```python
from build123d import *

# Parameters (mm, degrees)
F0_W     = 127
F0_H     = 76.2
F1_DEPTH = 50.8
F2_R     = 7.62
F3_W     = 7
F3_H     = 15.2537040412
F4_DEPTH = 16.4084
F4_TAPER = -3
F5_W     = 5
F5_H     = 4.0000001475
F6_DEPTH = 11.938
F6_TAPER = -3


with BuildPart() as f1:
    # F0 (on Front) → F1 (new body)
    with BuildSketch(Plane.XZ):
        Rectangle(F0_W, F0_H)
    extrude(amount=F1_DEPTH)

    # F2
    f2_edges = [f1.edges().sort_by_distance(p)[0] for p in [
        (0, -50.8, 38.1),
        (0, 0, 38.1),
        (0, -50.8, -38.1),
        (0, 0, -38.1),
    ]]
    fillet(f2_edges, radius=F2_R)

    # F3 (on face) → F4 (cut)
    with BuildSketch(Plane.YZ.offset(63.5)):
        with Locations((-38.6635434031, 24.1756830364)):
            Rectangle(F3_W, F3_H)
    extrude(amount=-F4_DEPTH, taper=F4_TAPER, mode=Mode.SUBTRACT)

    # F5 (on face) → F6 (cut)
    with BuildSketch(Plane.YZ.offset(63.5)):
        with Locations((-31.6249994836, 2.0000000738)):
            Rectangle(F5_W, F5_H)
    extrude(amount=-F6_DEPTH, taper=F6_TAPER, mode=Mode.SUBTRACT)


solid = f1.part
```
Check sheet for the modelled part. Datum: model origin and axes. Units: mm. A direction names the side the tool comes from. Round coordinates to 2 decimals unless told otherwise and drop trailing zeros. Write item = value, one per line. Start each with the question number.
1. Gauge pin test, flat ends, axial feed: pin 1 (1.5 mm diameter, centred on x = -47.5, y = -5.5, fed in from -Z); pin 2 (2.5 mm diameter, centred on y = -31.5, z = 2, fed in from +X). Record the tip position at first contact, or that the pin passes through.
2. Tool access check on faces 1 (the flat face through (47.092, -39, 24)), 2 (the flat face through (-1, -25, 38.1)). Record the directions out of +Z, -Z, +X, -X, +Y, -Y that give a thin tool (end or side, any length) a straight path to the whole face; none if there is none.
3. Release check for a two-part mould opening along Z. For faces 3 (the flat face through (63.5, -25, -1)), 4 (the flat face through (51.562, -32, 2)), 5 (the cylindrical face through (0.889, -2.291, -35.927)) record: pulls with the +Z half, pulls with the -Z half, needs draft (parallel to the pull), parting line crosses it, or undercut.
4. Scan lines: line 1 (X direction, y = -41, z = 25.5); line 2 (Y direction, x = 52, z = 31.5); line 3 (Z direction, x = 54, y = -35). Record each from-to range of solid material in increasing order. Write a range as [from, to].
Results found:
q1.pin_1 = -37.98
q1.pin_2 = 51.56
q2.face_1 = none
q2.face_2 = +Z, +X, -X, +Y, -Y
q3.face_3 = needs draft
q3.face_4 = undercut
q3.face_5 = pulls with the -Z half
q4.line_1 = [-63.5, 47.09]
q4.line_2 = [-50.73, -42.77], [-34.56, -0.07]
q4.line_3 = [-38.1, 16.05], [32.3, 38.1]
